Source: CAD feature listing. Evaluate the final solid. Frame: model axes, mm. Face numbers are marked on the shaded views. A direction names the side the tool comes from. Round coordinates to 2 decimals unless told otherwise and drop trailing zeros. Order: outer loops, then holes, each group sorted by start corner. A loop starts at its lowest first (then second) coordinate and runs counter-clockwise, first axis right, second up. Notation, with made-up numbers: (52, 18) -> (98, 18) arc R31 cw to (98, 43) -> close; hole circle Ø3 at (-2.75, -27.75). An arc over 180 degrees is marked (long way). Write item = value, one per line. Start each with the question number.
(1) Ray query, line 1 (X direction, y = -20, z = 18.6); line 2 (Z direction, x = -74.5, y = 35); line 3 (Z direction, x = -81, y = -19.5). Return the intervals inside material, ascending.
(2) Contact query for flat-ended pins moving along their axis: pin 1 Ø3 at (x, y) = (-91.42, 20) entering from -Z; pin 2 Ø7.5 at (x, z) = (-77, 15.5) entering from +Y; pin 3 Ø6.5 at (x, y) = (-92.69, 16.54) entering from -Z; pin 4 Ø1.5 at (y, z) = (-38.5, 5) entering from -X. Output: stop coordinate, or through.
(3) Cut plane C-C on z = 1.75. Return the cut outline in (x, y).
(4) Cut plane A-A on x = -77. Return the cut outline in (y, z).
(5) Cut plane D-D on z = 16.25. Return the cut outline in (x, y).
(6) Reachability of the marked faces 1, 2 and 3 from +Z, -Z, +X, -X, +Y, -Y: full face, straight path, thin tool, end or side. Return the list, or none.
(7) Draft query along Y for the marked faces 4, 5 and 6. Return one class per face: released by +Y, released by -Y, zero draft, split by the parting line, or undercut.
(8) Cut plane B-B on y = 0. Return the cut outline in (x, z), then the cut area to 3 significant figures.
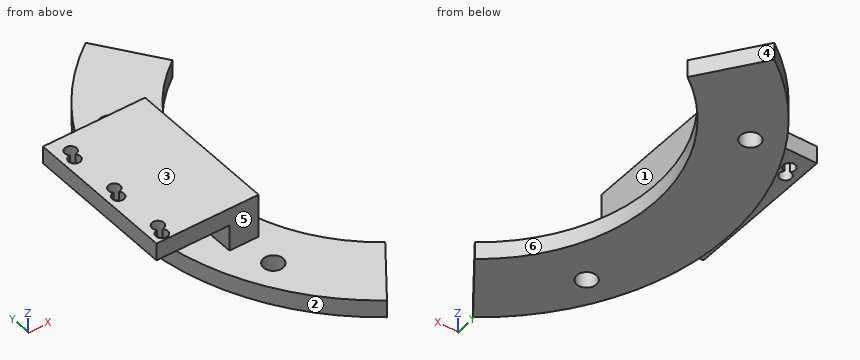
from build123d import *

# Parameters (mm, degrees)
SKETCH_1_R          = 85
SKETCH_1_R_2        = 60
EXTRUDE_1_DEPTH     = 6
SKETCH_2_R          = 3.35
CUT_EXTRUDE_1_DEPTH = 10
SKETCH_3_W          = 10
SKETCH_3_H          = 52
EXTRUDE_2_DEPTH     = 15
SKETCH_8_W          = 6
SKETCH_8_H          = 52
EXTRUDE_3_DEPTH     = 25
SKETCH_10_W         = 8.003334919
SKETCH_10_H         = 52
EXTRUDE_4_DEPTH     = 25
SKETCH_11_R         = 2
CUT_EXTRUDE_3_DEPTH = 25
CUT_EXTRUDE_4_DEPTH = 50
SKETCH_6_R          = 2
CUT_EXTRUDE_2_DEPTH = 20


with BuildPart() as part:
    # 草图1 → 凸台-拉伸1 (new body)
    with BuildSketch(Plane.XY):
        Circle(SKETCH_1_R)
        Circle(SKETCH_1_R_2, mode=Mode.SUBTRACT)
    extrude(amount=EXTRUDE_1_DEPTH)

    # 草图2 → 切除-拉伸1 (cut)
    with BuildSketch(Plane.XY.offset(6)):
        with Locations((0, 75)):
            Circle(SKETCH_2_R)
        with Locations((64.951905284, 37.5)):
            Circle(SKETCH_2_R)
        with Locations((64.951905284, -37.5)):
            Circle(SKETCH_2_R)
        with Locations((0, -75)):
            Circle(SKETCH_2_R)
        with Locations((-64.951905284, -37.5)):
            Circle(SKETCH_2_R)
        with Locations((-64.951905284, 37.5)):
            Circle(SKETCH_2_R)
    extrude(amount=-CUT_EXTRUDE_1_DEPTH, mode=Mode.SUBTRACT)

    # 草图3 → 凸台-拉伸2 (add)
    with BuildSketch(Plane.XY.offset(6)):
        with Locations((66.419532829, -0.009729533)):
            Rectangle(SKETCH_3_W, SKETCH_3_H)
        with Locations((-66.419532829, -0.009729533)):
            Rectangle(SKETCH_3_W, SKETCH_3_H)
    extrude(amount=EXTRUDE_2_DEPTH)

    # 草图8 → 凸台-拉伸3 (add)
    with BuildSketch(Plane.ZY.offset(71.419532829)):
        with Locations((18, -0.009729533)):
            Rectangle(SKETCH_8_W, SKETCH_8_H)
    extrude(amount=EXTRUDE_3_DEPTH)

    # 草图10 → 凸台-拉伸4 (add)
    with BuildSketch(Plane(origin=(71.419532829, 0, 0), x_dir=(0, 0, -1), z_dir=(1, 0, 0))):
        with Locations((-16.998332541, -0.009729533)):
            Rectangle(SKETCH_10_W, SKETCH_10_H)
    extrude(amount=EXTRUDE_4_DEPTH)

    # 草图11 → 切除-拉伸3 (cut)
    with BuildSketch(Plane.XY.offset(21)):
        with Locations((-91.419532829, 0)):
            Circle(SKETCH_11_R)
        with Locations((-91.419532829, 20)):
            Circle(SKETCH_11_R)
        with Locations(Location((91.419532829, 0, 0), (0, 0, 270))):
            Circle(SKETCH_11_R)
        with Locations(Location((91.419532829, 20, 0), (0, 0, 270))):
            Circle(SKETCH_11_R)
        with Locations((91.419532829, -20)):
            Circle(SKETCH_11_R)
        with Locations(Location((-91.419532829, -20, 0), (0, 0, 270))):
            Circle(SKETCH_11_R)
    extrude(amount=-CUT_EXTRUDE_3_DEPTH, mode=Mode.SUBTRACT)

    # 草图12 → 切除-拉伸4 (cut, symmetric)
    with BuildSketch(Plane.XY.offset(6)):
        with BuildLine():
            Line((-35, 48.733971724), (-49.583333333, 69.039793276))
            ThreePointArc((-49.583333333, 69.039793276), (-42.500689847, 73.611761034), (-35, 77.459666924))
            Line((-35, 77.459666924), (-35, 90))
            Line((-35, 90), (35, 90))
            Line((35, 90), (153.524849436, 90))
            Line((153.524849436, 90), (153.524849436, -90))
            Line((153.524849436, -90), (35, -90))
            Line((35, -90), (-35, -90))
            Line((-35, -90), (-35, -77.459666924))
            ThreePointArc((-35, -77.459666924), (-42.500689847, -73.611761034), (-49.583333333, -69.039793276))
            Line((-49.583333333, -69.039793276), (-35, -48.733971724))
            Line((-35, -48.733971724), (-35, 48.733971724))
        make_face()
    extrude(amount=CUT_EXTRUDE_4_DEPTH, both=True, mode=Mode.SUBTRACT)

    # 草图6 → 切除-拉伸2 (cut)
    with BuildSketch(Plane.XY.offset(26)):
        with Locations((92.689735177, -3.459773101)):
            Circle(SKETCH_6_R)
        with Locations((92.689735177, -23.459773101)):
            Circle(SKETCH_6_R)
        with Locations((92.689735177, 16.540226899)):
            Circle(SKETCH_6_R)
        with Locations((-92.689735177, -23.459773101)):
            Circle(SKETCH_6_R)
        with Locations((-92.689735177, -3.459773101)):
            Circle(SKETCH_6_R)
        with Locations((-92.689735177, 16.540226899)):
            Circle(SKETCH_6_R)
    extrude(amount=-CUT_EXTRUDE_2_DEPTH, mode=Mode.SUBTRACT)


solid = part.part
Evaluation:
q1.line_1 = -96.42 to -93.42, -89.42 to -61.42
q1.line_2 = 0 to 6
q1.line_3 = 0 to 6, 15 to 21
q2.pin_1 = through
q2.pin_2 = 25.99
q2.pin_3 = 15
q2.pin_4 = -76.16
q3.outline = (-49.58, -69.04) -> (-35, -48.73) arc R60 cw to (-35, 48.73) -> (-49.58, 69.04) arc R85 ccw to start; hole circle Ø6.7 at (-64.95, -37.5); hole circle Ø6.7 at (-64.95, 37.5)
q4.outline = (-36, 0) -> (36, 0) -> (36, 6) -> (-36, 6) -> close; (-26.01, 15) -> (25.99, 15) -> (25.99, 21) -> (-26.01, 21) -> close
q5.outline = (-96.42, -26.01) -> (-61.42, -26.01) -> (-61.42, 25.99) -> (-96.42, 25.99) -> close; hole (-92.78, -21.46) arc R2 ccw (long way) to (-91.32, -22) arc R2 ccw (long way) to start; hole (-92.78, -1.46) arc R2 ccw (long way) to (-91.32, -2) arc R2 ccw (long way) to start; hole (-92.78, 18.54) arc R2 ccw (long way) to (-91.32, 18) arc R2 ccw (long way) to start
q6.face_1 = +Z, +X, +Y, -Y
q6.face_2 = -Z, -X
q6.face_3 = +Z, +X, -X, +Y, -Y
q7.face_4 = released by +Y
q7.face_5 = released by -Y
q7.face_6 = undercut
q8.outline = (-96.42, 15) -> (-93.42, 15) -> (-93.42, 21) -> (-96.42, 21) -> close; (-89.42, 15) -> (-71.42, 15) -> (-71.42, 6) -> (-85, 6) -> (-85, 0) -> (-60, 0) -> (-60, 6) -> (-61.42, 6) -> (-61.42, 21) -> (-89.42, 21) -> close
q8.area = 426 mm^2
